Input: part model. Units: mm. Frame: model coordinates. Face numbers are marked on the shaded views. A direction names the side the tool comes from. Round coordinates to 2 decimals unless told otherwise and drop trailing zeros. Order: outer loops, then holes, each group sorted by start corner. A loop starts at its lowest first (then second) coordinate and runs counter-clockwise, first axis right, second up. Notation, with made-up numbers: (58, 17) -> (78, 17) arc R37 ccw to (78, 56) -> close; hole circle Ø9 at (45, 19). An arc over 180 degrees is marked (long way). Use a Markdown table: item, result.
from build123d import *

# Parameters (mm, degrees)
FILLET2_R  = 0.9
SKETCH2_W  = 5.6
SKETCH2_H  = 0.8
SLOT_DEPTH = 0.7


with BuildPart() as part:
    # BodySke → Base-Revolve (revolve)
    with BuildSketch(Plane.XY, mode=Mode.PRIVATE) as base_revolve_sk:
        Polygon((1.8, 1.5), (1.8, 2.8), (0, 2.642520406), (0, 0), (11.8, 0), (11.8, 1.5), align=None)
    revolve(base_revolve_sk.sketch.rotate(Axis((-25.4, 0, 0), (1, 0, 0)), 90), axis=Axis((-25.4, 0, 0), (1, 0, 0)))  # turned: the seam where the file's is

    # Fillet2
    fillet2_edges = [part.edges().sort_by_distance(p)[0] for p in [
        (0, 0, -2.642520406),
    ]]
    fillet(fillet2_edges, radius=FILLET2_R)

    # Sketch2 → Slot (cut)
    with BuildSketch(Plane(origin=(0, 0, 0), x_dir=(0, 0, -1), z_dir=(1, 0, 0))):
        Rectangle(SKETCH2_W, SKETCH2_H)
    extrude(amount=SLOT_DEPTH, mode=Mode.SUBTRACT)


solid = part.part
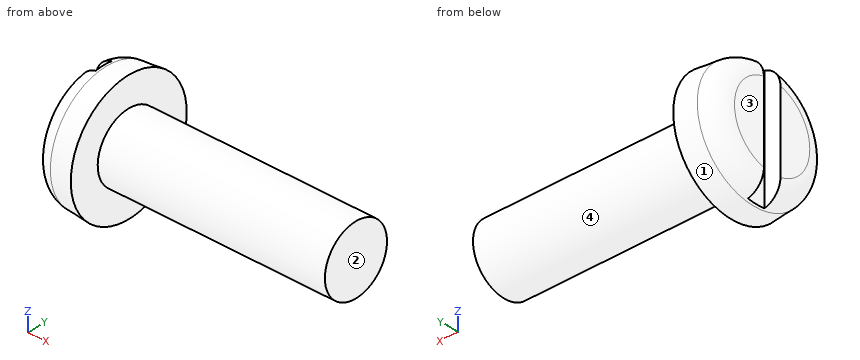
1) Cut plane B-B on y = 0. Return loops of the section in (x, z).
Results found:
| item | result |
|---|---|
| outline | (0.7, -2.7) arc R0.9 ccw to (0.82, -2.71) -> (1.8, -2.8) -> (1.8, -1.5) -> (11.8, -1.5) -> (11.8, 1.5) -> (1.8, 1.5) -> (1.8, 2.8) -> (0.82, 2.71) arc R0.9 ccw to (0.7, 2.7) -> close |
2) Pull-direction query (Z, two-part tool) for the marked faces 1 and 2; classes: +Z half, -Z half, draft (parallel to the pull), parting line (faces both ways), or undercut.
Results found:
| item | result |
|---|---|
| face 1 | parting line |
| face 2 | draft |
3) Pin query (flat end, axial travel): pin 1 Ø2 at (x, z) = (3, 0.5) entering from -Y; pin 2 Ø0.8 at (x, z) = (0, -0.5) entering from +Y; pin 3 Ø0.6 at (x, z) = (0, 1) entering from -Y. Return the tip coordinate at first contact, or that it passes through.
Results found:
| item | result |
|---|---|
| pin 1 | stops at y = -1.5 |
| pin 2 | stops at y = 2.53 |
| pin 3 | stops at y = -2.3 |
4) Cut plane A-A on z = 0. Return loops of the section in (x, y).
Results found:
| item | result |
|---|---|
| outline | (0, -1.82) arc R0.9 ccw to (0.82, -2.71) -> (1.8, -2.8) -> (1.8, -1.5) -> (11.8, -1.5) -> (11.8, 1.5) -> (1.8, 1.5) -> (1.8, 2.8) -> (0.82, 2.71) arc R0.9 ccw to (0, 1.82) -> (0, 0.4) -> (0.7, 0.4) -> (0.7, -0.4) -> (0, -0.4) -> close |
5) Set-up query: the marked faces 3 and 4. Return all of +Z, -Z, +X, -X, +Y, -Y with unobstructed straight access to the full face (end or side cutting, diameter ignored); none if empty.
Results found:
| item | result |
|---|---|
| face 3 | +Z, -Z, -X, +Y, -Y |
| face 4 | +X |
6) Cut plane C-C on x = 7.75. Return loops of the section in (y, z).
Results found:
| item | result |
|---|---|
| outline | circle Ø3 at (0, 0) |
7) Line query: L1, parallel to X at y = 1.2, z = 1.1; L2, parallel to X at y = 0.2, z = 1.75; L3, parallel to Y at x = 9.25, z = 0.55. Output: solid intervals per line, ascending. Write a range as [from, to].
Results found:
| item | result |
|---|---|
| L1 | x = [0, 1.8] |
| L2 | x = [0.7, 1.8] |
| L3 | y = [-1.4, 1.4] |
